Verification items for the finished model (mm, model axes). Face numbers are marked on the shaded views. A direction names the side the tool comes from. Coordinates: 2 decimals unless noted, no trailing zeros. Loops run counter-clockwise (first coordinate to the right, second up) from the corner with the lowest first, then second, coordinate; pieces in that order, holes last. Notation, with made-up numbers: (27.5, -38) -> (43.5, -38) arc R16 ccw to (43.5, -33) -> close; hole circle Ø5 at (52, 4.5). An arc over 180 degrees is marked (long way). Answer as a JSON object with one key per item and string values. Group by question number.
Q1. Cross-section at C-C on z = -125.5. Record the boundary of the cut face in (x, y).
Q2. Release check for a two-part mould opening along Z. For the marked faces 1, 2, 3 and 4 record: released by +Z, released by -Z, zero draft, split by the parting line, or undercut.
Q3. Cross-section at A-A on y = 76. Record the boundary of the cut face in (x, z), and give its area (3 significant figures).
Q4. Cross-section at B-B on x = 94.5. Record the boundary of the cut face in (y, z).
Q5. Set-up check for the marked faces 5 and 6: record each of +Z, -Z, +X, -X, +Y, -Y from which the full face is reachable in a straight line by a thin tool's end or side.
Q6. Scan lines: L1, parallel to Z at x = 13, y = 25; L2, parallel to Y at x = 66.5, z = -22. Record each from-to range of solid material in increasing order.
Q7. Gauge pin test, flat ends, axial feed: pin 1 Ø5 at (y, z) = (2, -86) entering from -X; pin 2 Ø1.4 at (y, z) = (69.5, -168) entering from +X; pin 3 Ø1.2 at (x, z) = (152.5, -3.5) entering from +Y. Record the tip position at first contact, or that the pin passes through.
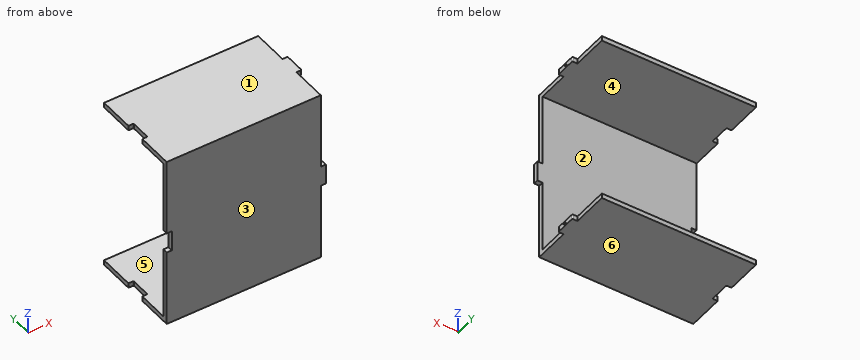
Autodesk Inventor part; units mm, degrees
ref_plane "YZ Plane" through (0, 0, 0) normal (1, 0, 0) x (0, 1, 0)
ref_plane "XZ Plane" through (0, 0, 0) normal (0, 1, 0) x (-1, 0, 0)
ref_plane "XY Plane" through (0, 0, 0) normal (0, 0, 1) x (1, 0, 0)
sketch "Sketch1" plane through (0, 0, 0) normal (0, 1, 0) x (-1, 0, 0)
  line L0 (0, 0) -> (-150, 0)
  line L1 (0, -170) -> (-150, -170)
  line L2 (-150, -170) -> (-150, -95)
  line L3 (-150, -95) -> (-155, -95)
  line L4 (-155, -95) -> (-155, -75)
  line L5 (-155, -75) -> (-150, -75)
  line L6 (-150, -75) -> (-150, 0)
  line L7 (0, -170) -> (0, -95)
  line L8 (0, -95) -> (-5, -95)
  line L9 (-5, -95) -> (-5, -75)
  line L10 (-5, -75) -> (0, -75)
  line L11 (0, -75) -> (0, 0)
  dimension "d0" = 150
  dimension "d1" = 170
  dimension "d2" = 5
  dimension "d3" = 5
  dimension "d4" = 75
  dimension "d5" = 75
  dimension "d6" = 20
  dimension "d9" = 0
  dimension "d10" = 75
  dimension "d11" = 5
  dimension "d12" = 75
  dimension "d13" = 20
  dimension "d14" = 150
  dimension "d15" = 0
extrude "Extrusion1" add sketch "Sketch1" along normal blind 4.7625
sketch "Sketch2" plane through (0, 4.7625, 0) normal (0, 1, 0) x (1, 0, 0)
  line L0 (0, 0) -> (150, 0)
  line L1 (0, 0) -> (150, 0)
  line L2 (150, 0) -> (150, 4.7625)
  line L3 (150, 0) -> (150, 75)
  line L4 (150, 4.7625) -> (0, 4.7625)
  line L5 (0, 75) -> (0, 0)
  line L6 (0, 0) -> (0, 4.7625)
  line L7 (150, 170) -> (0, 170)
  line L8 (0, 170) -> (150, 170)
  line L9 (150, 170) -> (150, 165.2375)
  line L10 (150, 95) -> (150, 170)
  line L11 (150, 165.2375) -> (0, 165.2375)
  line L12 (0, 170) -> (0, 95)
  line L13 (0, 170) -> (0, 165.2375)
  dimension "d18" = 4.7625
  dimension "d19" = 4.7625
extrude "Extrusion2" add sketch "Sketch2" along normal blind 85.2375
sketch "Sketch3" plane through (0, 0, 0) normal (0, 0, 1) x (1, 0, 0)
  line L0 (0, 0) -> (0, 90)
  line L1 (0, 55) -> (5, 55)
  line L2 (5, 55) -> (5, 35)
  line L3 (5, 35) -> (0, 35)
  line L4 (0, 55) -> (0, 35)
  line L5 (0, 90) -> (150, 90)
  line L6 (0, 0) -> (150, 0)
  dimension "d22" = 20
  dimension "d23" = 5
  dimension "d24" = 35
  dimension "d25" = 35
extrude "Extrusion3" cut sketch "Sketch3" against normal blind 4.7625
sketch "Sketch4" plane through (150, 0, -170) normal (0, 0, -1) x (-1, 0, 0)
  line L0 (150, 0) -> (150, 90)
  line L1 (150, 35) -> (145, 35)
  line L2 (145, 35) -> (145, 55)
  line L3 (145, 55) -> (150, 55)
  line L4 (150, 55) -> (150, 35)
  line L5 (0, 90) -> (150, 90)
  line L6 (0, 0) -> (150, 0)
  dimension "d28" = 20
  dimension "d29" = 5
  dimension "d30" = 35
  dimension "d31" = 35
extrude "Extrusion4" cut sketch "Sketch4" against normal blind 4.7625
sketch "Sketch5" plane through (0, 0, 0) normal (0, 0, 1) x (1, 0, 0)
  line L0 (150, 0) -> (150, 90)
  line L1 (150, 55) -> (155, 55)
  line L2 (155, 55) -> (155, 35)
  line L3 (155, 35) -> (150, 35)
  line L4 (150, 35) -> (150, 55)
  line L5 (0, 0) -> (150, 0)
  line L6 (0, 90) -> (150, 90)
  dimension "d34" = 20
  dimension "d35" = 5
  dimension "d36" = 35
  dimension "d37" = 35
extrude "Extrusion5" add sketch "Sketch5" against normal blind 4.7625
sketch "Sketch6" plane through (150, 0, -170) normal (0, 0, -1) x (-1, 0, 0)
  line L0 (0, 55) -> (-5, 55)
  line L1 (0, 55) -> (-5, 55)
  line L2 (-5, 55) -> (-5, 35)
  line L3 (0, 4.7625) -> (0, 35)
  line L4 (-5, 35) -> (0, 35)
  line L5 (0, 35) -> (0, 55)
  point P0 (150, 0)
extrude "Extrusion6" add sketch "Sketch6" against normal blind 4.7625
fillet "Fillet1" radius 1 4 edges at (5, 35, -167.6188) (5, 55, -167.6188) (5, 55, -2.3813) (5, 35, -2.3813)
fillet "Fillet2" radius 1 4 edges at (155, 55, -2.3813) (155, 35, -2.3813) (155, 55, -167.6188) (155, 35, -167.6188)
hole "Hole1" at (155, 45.4891, -2.2612) direction (-1, 0, 0) diameter 2.5 depth 5 tip angle 118
hole "Hole2" at (155, 44.4165, -167.8579) direction (-1, 0, 0) diameter 2.5 depth 5 tip angle 118
properties part number "OpticalDeviceLensPart (1)"
Computed values:
{
 "1": {"outline": "(0, 0) -> (150, 0) -> (150, 4.76) -> (0, 4.76) -> close"},
 "2": {"face 1": "released by +Z", "face 2": "undercut", "face 3": "zero draft", "face 4": "undercut"},
 "3": {"outline": "(0, -170) -> (150, -170) -> (150, -165.24) -> (0, -165.24) -> close; (0, -4.76) -> (150, -4.76) -> (150, 0) -> (0, 0) -> close", "area": "1,430 mm²"},
 "4": {"outline": "(0, -170) -> (90, -170) -> (90, -165.24) -> (4.76, -165.24) -> (4.76, -4.76) -> (90, -4.76) -> (90, 0) -> (0, 0) -> close"},
 "5": {"face 5": "+X, -X, +Y", "face 6": "-Z, +X, -X, +Y, -Y"},
 "6": {"L1": "z = -170 to -165.24, -4.76 to 0", "L2": "y = 0 to 4.76"},
 "7": {"pin 1": "stops at x = 5", "pin 2": "stops at x = 150", "pin 3": "stops at y = 55"}
}
